The drawing under review shows one solid part. Ordinate dimensions are in mm from its lowest x, y, z. A direction names the side the tool comes from. Coordinates: 2 decimals unless noted, no trailing zeros. Write each loop counter-clockwise with the first axis right and the second up, starting at its lowest first coordinate (ties: lowest second). Pieces come first, ordered by that corner, then holes.
Q1. Add section D-D, the plane y = 38. Give the boundary of the cut face in (x, z).
Q2. Clearance check with flat-ended pins moving along their axes: pin 1 Ø1 at (x, y) = (26, 5.5) entering from -Z; pin 2 Ø3 at (x, z) = (15, 1.5) entering from +Y; pin 3 Ø3.5 at (x, y) = (38, 20.5) entering from +Z. State where each tip first meets the part, or that it passes through.
Q3. Add section A-A, the plane y = 20.5. Give the boundary of the cut face in (x, z).
Q4. Machinability: for the marked faces 1, 2 and 3, which of the approach directions +Z, -Z, +X, -X, +Y, -Y give a long, thin tool a straight path to every point of the face, cutting with its end or side? Answer none if there is none.
Q5. To check wall thickness, follow probe 1 along Y at (x, z) = (20.5, 4.25); probe 2 along X at (y, z) = (8.5, 2.5) (1 decimal); probe 3 along X at (y, z) = (7.5, 3). State the ranges of each line that lie inside material, in increasing order.
Q6. Add section C-C, the plane z = 3.75. Give the number of separate pieces and of enclosed holes in the cut face, plus the area to 3 significant figures.
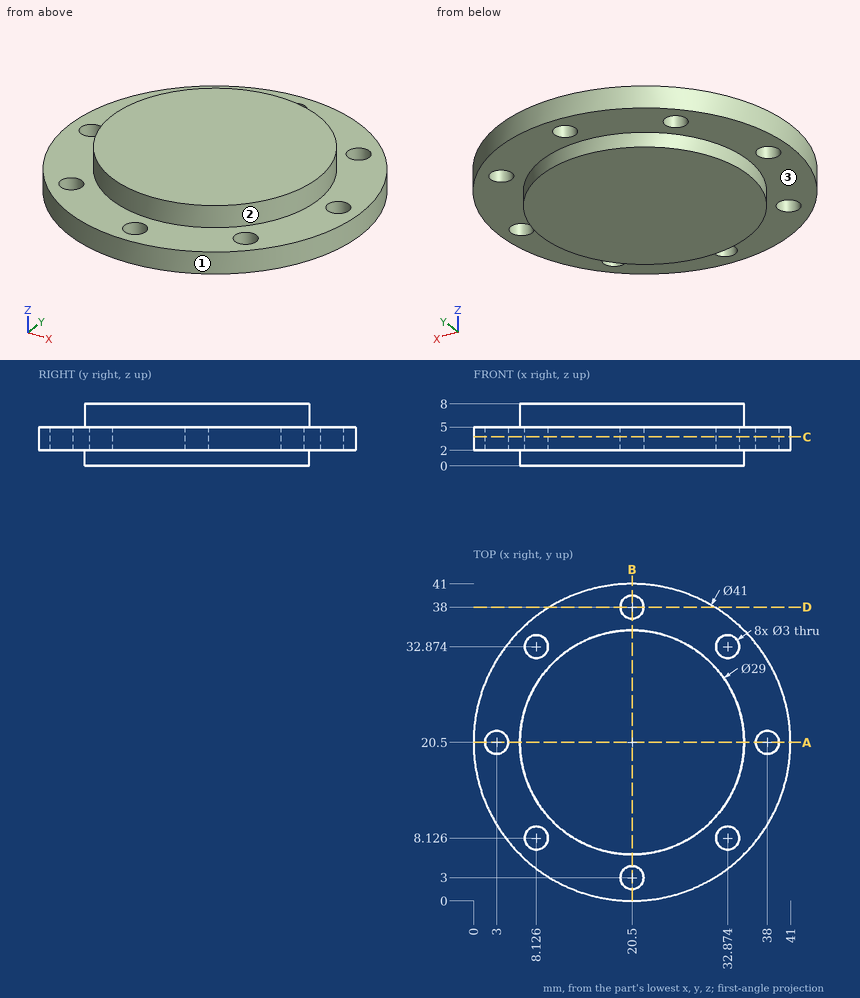
Here are the results:
1. outline: (9.82, 2) - (19, 2) - (19, 5) - (9.82, 5) - close; (22, 2) - (31.18, 2) - (31.18, 5) - (22, 5) - close
2. pin 1: stops at z = 2
2. pin 2: stops at y = 40.59
2. pin 3: stops at z = 5
3. outline: (0, 2) - (1.5, 2) - (1.5, 5) - (0, 5) - close; (4.5, 2) - (6, 2) - (6, 0) - (35, 0) - (35, 2) - (36.5, 2) - (36.5, 5) - (35, 5) - (35, 8) - (6, 8) - (6, 5) - (4.5, 5) - close; (39.5, 2) - (41, 2) - (41, 5) - (39.5, 5) - close
4. face 1: +Z, -Z
4. face 2: +Z
4. face 3: -Z
5. probe 1: y = 0 to 1.5, 4.5 to 36.5, 39.5 to 41
5. probe 2: x = 3.9 to 6.7, 9.6 to 31.4, 34.3 to 37.1
5. probe 3: x = 4.65 to 6.76, 9.49 to 31.51, 34.24 to 36.35
6. separate pieces: 1
6. enclosed holes: 8
6. area: 1,260 mm2
